Autodesk Inventor part; units mm, degrees
ref_plane "YZ Plane" through (0, 0, 0) normal (1, 0, 0) x (0, 1, 0)
ref_plane "XZ Plane" through (0, 0, 0) normal (0, 1, 0) x (-1, 0, 0)
ref_plane "XY Plane" through (0, 0, 0) normal (0, 0, 1) x (1, 0, 0)
sketch "Эскиз1" plane through (0, 0, 0) normal (1, 0, 0) x (0, 1, 0)
  line L0 (0, 0) -> (-5, 0)
  line L1 (-5, 0) -> (-5, -15)
  line L2 (-5, -15) -> (0, -15)
  line L3 (0, -15) -> (0, 0)
  circle A0 centre (0, 0) radius 5
  circle A1 centre (0, -15) radius 5
  circle A2 centre (0, 0) radius 0.5
  circle A3 centre (0, -15) radius 0.5
  point P0 (0, -5)
  point P1 (0, -10)
  dimension "d0" = 5
  dimension "d1" = 15
  dimension "d4" = 1
  dimension "d5" = 1
extrude "Выдавливание1" add sketch "Эскиз1" along normal blind 40 contours A2 L3 A0 L0 | L0 A0 L3 A2 | A0 L3 A1 L1 | A1 L3 A3 L2 | L2 A3 L3 A1
sketch "Эскиз2" plane through (0, 0, -5) normal (0, 1, 0) x (1, 0, 0)
  line L0 (0, 0) -> (40, 0)
  line L1 (0, -10) -> (40, -10)
  line L2 (10, 0) -> (30, 0)
  line L3 (30, 0) -> (30, -10)
  line L4 (30, -10) -> (10, -10)
  line L5 (10, -10) -> (10, 0)
  line L6 (0, 5) -> (0, 0)
  line L7 (40, 5) -> (40, 0)
  point P0 (0, -5)
  dimension "d6" = 10
  dimension "d7" = 10
extrude "Выдавливание2" cut sketch "Эскиз2" along normal mid plane 10
sketch "Эскиз3" plane through (0, 0, -5) normal (0, 1, 0) x (1, 0, 0)
  line L0 (0, 5) -> (40, 5)
  line L1 (0, 15) -> (40, 15)
  line L2 (10, 5) -> (0, 5)
  line L3 (0, 5) -> (0, 15)
  line L4 (0, 15) -> (10, 15)
  line L5 (10, 15) -> (10, 5)
  line L6 (40, 5) -> (40, 15)
  line L7 (30, 5) -> (40, 5)
  line L8 (40, 5) -> (40, 15)
  line L9 (40, 15) -> (30, 15)
  line L10 (30, 15) -> (30, 5)
  line L11 (40, 5) -> (40, 0)
  line L12 (0, 5) -> (0, 0)
  point P0 (0, -5)
  point P1 (40, 10)
  point P2 (10, 15)
  dimension "d10" = 10
  dimension "d11" = 10
extrude "Выдавливание3" cut sketch "Эскиз3" against normal mid plane 10 contours L3 L1 L5 L0 | L10 L1 L6 L0
sketch "Эскиз10" plane through (10, 0, -5) normal (0, 1, 0) x (1, 0, 0)
  line L0 (2, 1) -> (18, 1)
  line L1 (18, 1) -> (18, 4)
  line L2 (18, 4) -> (2, 4)
  line L3 (2, 4) -> (2, 1)
  line L4 (20, -10) -> (20, 0)
  line L5 (0, 5) -> (0, 15)
  line L6 (0, 0) -> (20, 0)
  line L7 (-10, 5) -> (0, 5)
  point P0 (-10, -5)
  point P1 (20, -5)
  point P2 (0, 10)
  dimension "d37" = 2
  dimension "d38" = 2
  dimension "d39" = 1
  dimension "d40" = 1
extrude "Выдавливание9" cut sketch "Эскиз10" against normal blind 2
properties part number "фаланга гусеницы"
Read the model definition and answer for the solid it produces. Units are mm, in the model's axes. A direction names the side the tool comes from. Round coordinates to 2 decimals unless told otherwise and drop trailing zeros. Write each loop counter-clockwise with the first axis right and the second up, starting at its lowest first coordinate (ties: lowest second). Pieces come first, ordered by that corner, then holes. Notation, with made-up numbers: (-14.5, 12.25) - (8.5, 12.25) arc R9 ccw to (8.5, 28.25) - close; hole circle Ø4 at (-20, 7.25). An arc over 180 degrees is marked (long way). Use CSV: the item, a comma, the result in double quotes.
Q1. Find section C-C, the plane x = 19. Write down the section's boundary in (y, z).
Values:
outline,"(-5, -15) arc R5 ccw (long way) to (0, -10) - (0, -9) - (-2, -9) - (-2, -6) - (0, -6) - (0, -5) - (-5, -5) - close; hole circle Ø1 at (0, -15)"
Q2. Find section A-A, the plane z = -3. Write down the section's boundary in (x, y).
Values:
outline,"(0, -5) - (10, -5) - (10, 4) - (0, 4) - close; (30, -5) - (40, -5) - (40, 4) - (30, 4) - close"
Q3. Find section B-B, the plane x = 37.5. Write down the section's boundary in (y, z).
Values:
outline,"(-5, -10) - (0, -10) - (0, -5) arc R5 ccw (long way) to (-5, 0) - close; hole circle Ø1 at (0, 0)"
Q4. Find section D-D, the plane z = 1.5. Write down the section's boundary in (x, y).
Values:
outline,"(0, -4.77) - (10, -4.77) - (10, 4.77) - (0, 4.77) - close; (30, -4.77) - (40, -4.77) - (40, 4.77) - (30, 4.77) - close"
Q5. Straight lines are drawn through the part: line 1 along X through (y, z) = (-1.5, 3.5); line 2 along Y through (x, z) = (21.25, -15); line 3 along X through (y, z) = (-1.5, -6.5). For each, find the intervals that lie inside material, in ascending order.
Values:
line 1,"x = 0 to 10, 30 to 40"
line 2,"y = -5 to -0.5, 0.5 to 5"
line 3,"x = 0 to 12, 28 to 40"
Q6. Determine the mould class of faces 5 (the cylindrical face through (4.93, -0.108, 0.488)), 6 (the flat face through (10, 0, -1)), 7 (the flat face through (19.7, 0, -9.2)) for opening direction Y: +Y half, -Y half, draft (parallel to the pull), parting line (faces both ways), or undercut.
Values:
face 5,"undercut"
face 6,"draft"
face 7,"+Y half"
Q7. Each of these flat-tipped pins is pushed along its axis until it touches: pin 1 Ø1.5 at (x, y) = (7, -2.5) entering from -Z; pin 2 Ø1 at (x, z) = (10.5, -12) entering from +Y; pin 3 Ø1.5 at (x, y) = (19, -3) entering from +Z. Where does it stop, or does it pass through?
Values:
pin 1,"stops at z = -10"
pin 2,"stops at y = 4.33"
pin 3,"stops at z = -5"
Q8. A tool of negligible diameter and unlimited length cuts with its end or side. For faces 1 (the flat face through (10, -1, -15)), 2 (the flat face through (28, -1, -7)), 3 (the flat face through (20, -3, -5)), 4 (the flat face through (35, -2, -10)), from which of +Z, -Z, +X, -X, +Y, -Y can it reach the whole face along a straight path? Write none if from no direction.
Values:
face 1,"-Z, -X, +Y, -Y"
face 2,"+Y"
face 3,"+Z, +Y, -Y"
face 4,"-Z, +X, +Y, -Y"
